from build123d import *

# Parameters (mm, degrees)
CROQUIS1_W              = 200
CROQUIS1_H              = 200
SALIENTE_EXTRUIR1_DEPTH = 50
CROQUIS2_W              = 25
CROQUIS2_H              = 25
SALIENTE_EXTRUIR2_DEPTH = 875


with BuildPart() as part:
    # Croquis1 → Saliente-Extruir1 (new body)
    with BuildSketch(Plane(origin=(0, 0, 0), x_dir=(1, 0, 0), z_dir=(0, 1, 0))):
        with Locations((100, 100)):
            Rectangle(CROQUIS1_W, CROQUIS1_H)
    extrude(amount=SALIENTE_EXTRUIR1_DEPTH)

    # Croquis2 → Saliente-Extruir2 (add)
    with BuildSketch(Plane.XZ):
        with Locations((12.5, -12.5)):
            Rectangle(CROQUIS2_W, CROQUIS2_H)
        with Locations((187.5, -12.5)):
            Rectangle(CROQUIS2_W, CROQUIS2_H)
        with Locations((12.5, -187.5)):
            Rectangle(CROQUIS2_W, CROQUIS2_H)
        with Locations((187.5, -187.5)):
            Rectangle(CROQUIS2_W, CROQUIS2_H)
    extrude(amount=SALIENTE_EXTRUIR2_DEPTH)


solid = part.part
Input: part model. Units: mm. Frame: model coordinates. A direction names the side the tool comes from. Round coordinates to 2 decimals unless told otherwise and drop trailing zeros. Loops run counter-clockwise (first coordinate to the right, second up) from the corner with the lowest first, then second, coordinate; pieces in that order, holes last. Notation, with made-up numbers: (2, -23.75) -> (53, -23.75) arc R15 ccw to (53, 5.25) -> close; hole circle Ø2 at (34.25, 54). An arc over 180 degrees is marked (long way). Answer as a JSON object with one key per item and string values. Group by question number.
1) Section query B-B on x = 151. Output: boundary loops of the cut face in (y, z).
2) Section query A-A on y = -501.5. Output: boundary loops of the cut face in (x, z).
3) Pin query (flat end, axial travel): pin 1 (2 mm diameter, centred on x = 26.5, y = -533.5, fed in from +Z); pin 2 (5 mm diameter, centred on x = 139, z = -117, fed in from -Y). Return the tip coordinate at first contact, or that it passes through.
4) Draft query along Z for faces 1 (the flat face through (18, -308, 0)), 2 (the flat face through (0, -308, -182)), 3 (the flat face through (12, -431, -175)). Return one class per face: +Z half, -Z half, draft (parallel to the pull), parting line (faces both ways), or undercut.
5) Ray query, L1, parallel to X at y = -505, z = -8.5; L2, parallel to Z at x = 24, y = -485; L3, parallel to Y at x = 115, z = -35. Return the intervals inside material, ascending.
6) Reachability of faces 4 (the flat face through (12, -431, -25)), 5 (the flat face through (200, -380, -181)), 6 (the flat face through (25, -431, -188)) from +Z, -Z, +X, -X, +Y, -Y: full face, straight path, thin tool, end or side. Return the list, or none.
7) Section query C-C on z = -88.5. Output: boundary loops of the cut face in (x, y).
Reply:
{
 "1": {"outline": "(0, -200) -> (50, -200) -> (50, 0) -> (0, 0) -> close"},
 "2": {"outline": "(0, -200) -> (25, -200) -> (25, -175) -> (0, -175) -> close; (0, -25) -> (25, -25) -> (25, 0) -> (0, 0) -> close; (175, -200) -> (200, -200) -> (200, -175) -> (175, -175) -> close; (175, -25) -> (200, -25) -> (200, 0) -> (175, 0) -> close"},
 "3": {"pin 1": "passes through", "pin 2": "stops at y = 0"},
 "4": {"face 1": "+Z half", "face 2": "draft", "face 3": "undercut"},
 "5": {"L1": "x = 0 to 25, 175 to 200", "L2": "z = -200 to -175, -25 to 0", "L3": "y = 0 to 50"},
 "6": {"face 4": "+X, -X, -Y", "face 5": "+Z, -Z, +X, +Y, -Y", "face 6": "+Z, -Z, -Y"},
 "7": {"outline": "(0, 0) -> (200, 0) -> (200, 50) -> (0, 50) -> close"}
}
